Can you work these out from the drawing? Everything is in mm from the part's minimum corner. Coordinates: 2 decimals unless noted, no trailing zeros. Order: outer loops, then holes, each group sorted by start corner. A loop starts at its lowest first (then second) coordinate and runs counter-clockwise, first axis right, second up. Notation, with made-up numbers: M -38.5,-35.75 L -9.5,-35.75 A21 ccw -9.5,-30.75 Z; hole C -31,59 d9. An arc over 180 degrees is marked long. Answer as a JSON object with one key per item and string values.
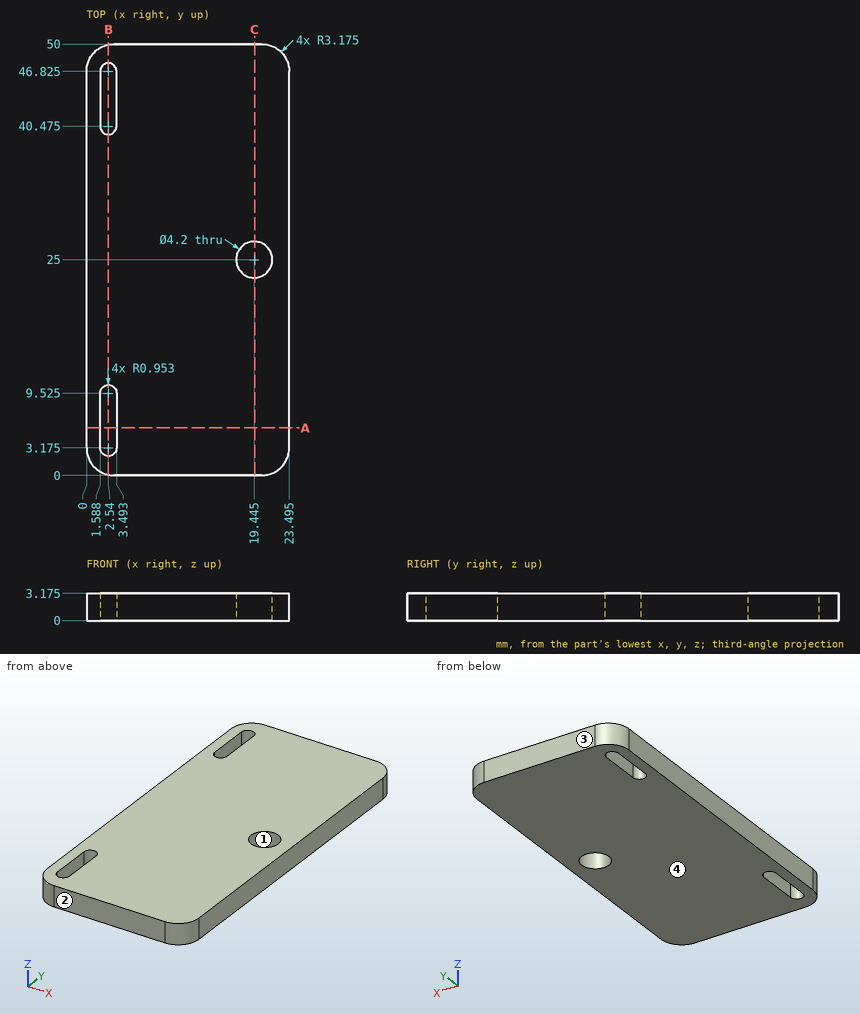
Item 1: If we mould it in two halves opening along Y, with no side actions, what happens to the marked faces 1, 2, 3 and 4? For each: pulls with the +Y half, pulls with the -Y half, needs draft (parallel to the pull), parting line crosses it, or undercut.
Answers follow:
{"face 1": "undercut", "face 2": "pulls with the -Y half", "face 3": "pulls with the +Y half", "face 4": "needs draft"}
Item 2: Please list where these lines run through material, in increasing order: line 1 (X direction, y = 42, z = 2.6) (1 decimal); line 2 (Y direction, x = 1.75, z = 0.65) (1 decimal); line 3 (X direction, y = 24, z = 1.85) (1 decimal).
Answers follow:
{"line 1": "x = 0 to 1.6, 3.5 to 23.5", "line 2": "y = 0.3 to 2.6, 10.1 to 39.9, 47.4 to 49.7", "line 3": "x = 0 to 17.6, 21.3 to 23.5"}
Item 3: I want a section at C-C, the plane x = 19.5. Write out the boundary of the cut face in (y, z) (1 decimal).
Answers follow:
{"outline": "M 0,0 L 22.9,0 L 22.9,3.2 L 0,3.2 Z; M 27.1,0 L 50,0 L 50,3.2 L 27.1,3.2 Z"}
Item 4: I want a section at B-B, the plane x = 2.54. Write out the boundary of the cut face in (y, z) (1 decimal).
Answers follow:
{"outline": "M 0.1,0 L 2.2,0 L 2.2,3.2 L 0.1,3.2 Z; M 10.5,0 L 39.5,0 L 39.5,3.2 L 10.5,3.2 Z; M 47.8,0 L 49.9,0 L 49.9,3.2 L 47.8,3.2 Z"}
Item 5: I want a section at A-A, the plane y = 5.5. Write out the boundary of the cut face in (x, z) (1 decimal).
Answers follow:
{"outline": "M 0,0 L 1.6,0 L 1.6,3.2 L 0,3.2 Z; M 3.5,0 L 23.5,0 L 23.5,3.2 L 3.5,3.2 Z"}
Item 6: I'm going to push a flat-ended pin straight in: pin 1 (2.5 mm diameter, centred on x = 19.445, y = 25, fed in from +Z). Where does the tip first touch, or does it pass through?
Answers follow:
{"pin 1": "passes through"}
